The drawing under review shows one solid part. Ordinate dimensions are in mm from its lowest x, y, z. A direction names the side the tool comes from. Coordinates: 2 decimals unless noted, no trailing zeros. Write each loop counter-clockwise with the first axis right and the second up, starting at its lowest first coordinate (ties: lowest second). Pieces come first, ordered by that corner, then holes.
Q1. Add section B-B, the plane z = 11.5. Give the boundary of the cut face in (x, y) (1 decimal).
Q2. Clearance check with flat-ended pins moving along their axes: pin 1 Ø10 at (y, z) = (5.5, 34.5) entering from -X; pin 2 Ø5 at (y, z) = (7.5, 40.5) entering from -X (1 decimal); pin 3 Ø17.5 at (x, z) = (140.79, 13.33) entering from -Y; pin 4 Ø2 at (y, z) = (19.5, 68.5) entering from -X. State where each tip first meets the part, or that it passes through.
Q3. Machinability: for the marked faces 5 and 6, which of the approach directions +Z, -Z, +X, -X, +Y, -Y give a long, thin tool a straight path to every point of the face, cutting with its end or side? Answer none if there is none.
Q4. The part is to be moulded in two halves that separate along Z. For the marked faces 1, 2, 3 and 4, say which applies: +Z half, -Z half, draft (parallel to the pull), parting line (faces both ways), or undercut.
Q5. To check wall thickness, follow probe 1 along X at (y, z) = (21.25, 77) (1 decimal); probe 2 along Y at (x, z) = (128, 47); probe 3 along X at (y, z) = (14.25, 46.5) (1 decimal). State the ranges of each line that lie inside material, in increasing order.
Q6. Add section C-C, the plane x = 84.5. Give the boundary of the cut face in (y, z), plus the area to 3 significant figures.
Q7. Add section D-D, the plane y = 20.5. Give the number of separate pieces and of enclosed holes in the cut face, plus the area to 3 significant figures.
Q8. Add section A-A, the plane z = 53. Give the boundary of the cut face in (x, y), plus the area to 3 significant figures.
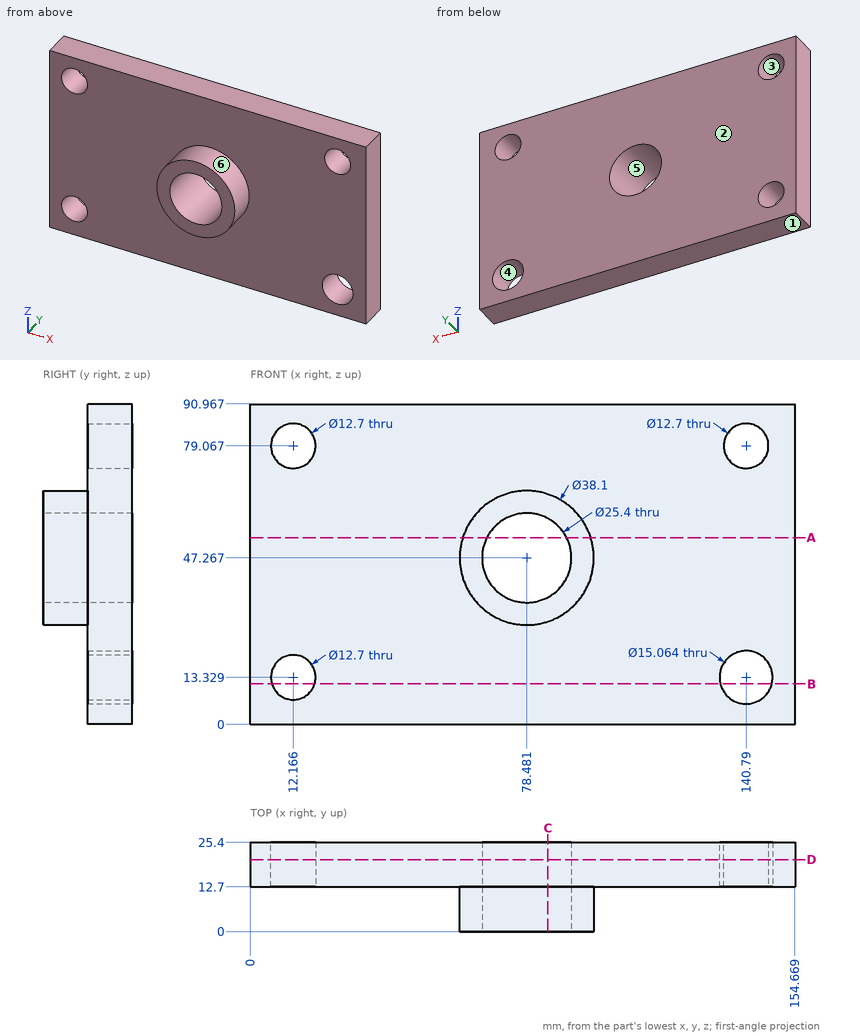
Here are the results:
1. outline: (0, 12.7) - (6.1, 12.7) - (6.1, 25.4) - (0, 25.4) - close; (18.2, 12.7) - (133.5, 12.7) - (133.5, 25.4) - (18.2, 25.4) - close; (148.1, 12.7) - (154.7, 12.7) - (154.7, 25.4) - (148.1, 25.4) - close
2. pin 1: stops at x = 61.09
2. pin 2: stops at x = 59.9
2. pin 3: stops at y = 12.7
2. pin 4: stops at x = 0
3. face 5: +Y, -Y
3. face 6: -Y
4. face 1: -Z half
4. face 2: draft
4. face 3: undercut
4. face 4: undercut
5. probe 1: x = 0 to 6.2, 18.2 to 134.8, 146.8 to 154.7
5. probe 2: y = 12.7 to 25.4
5. probe 3: x = 0 to 65.8, 91.2 to 154.7
6. outline: (0, 29.19) - (12.7, 29.19) - (12.7, 0) - (25.4, 0) - (25.4, 36.08) - (0, 36.08) - close; (0, 58.45) - (25.4, 58.45) - (25.4, 90.97) - (12.7, 90.97) - (12.7, 65.34) - (0, 65.34) - close
6. area: 1,050 mm2
7. separate pieces: 1
7. enclosed holes: 5
7. area: 13,000 mm2
8. outline: (0, 12.7) - (60.31, 12.7) - (60.31, 0) - (67.15, 0) - (67.15, 25.4) - (0, 25.4) - close; (89.81, 0) - (96.65, 0) - (96.65, 12.7) - (154.67, 12.7) - (154.67, 25.4) - (89.81, 25.4) - close
8. area: 1,850 mm2
